Geometry check sheet. Reference: the model listing, model coordinates, mm. A direction names the side the tool comes from. Round coordinates to 2 decimals unless told otherwise and drop trailing zeros. Loops run counter-clockwise (first coordinate to the right, second up) from the corner with the lowest first, then second, coordinate; pieces in that order, holes last. Notation, with made-up numbers: (50, -4) - (103, -4) arc R15 cw to (103, 24) - close; hole circle Ø6 at (-30.75, 88.5). An arc over 180 degrees is marked (long way). Answer in a Markdown table with one row per item. Add a question column.
```python
from build123d import *

# Parameters (mm, degrees)
F3_R = 4.3853298938


with BuildPart() as f1:
    # F0 (on Front) → F1 (revolve)
    with BuildSketch(Plane.XZ):
        Polygon((44.2099806775, 105.9490938586), (45.2899709793, 125.555711587), (44.2724308081, 125.555711587), (37.4149333342, 1.0616940765), (0, 1.0616940765), (0, 0), (35.287540406, 0), (35.287540406, -1.444288413), (38.2944366026, -1.444288413), (40.1810593803, 32.8062891499), (40.531485917, 39.1680862292), (43.8607326026, 99.6086910919), align=None)
    revolve(axis=Axis((0, 0, 69.7766542435), (0, 0, 1)))

    # F4: sweep along a path in F0
    with BuildLine(Plane.XZ) as f4_path:
        add(Plane.XZ * Edge.make_bspline(
            [(44.2099806775, 105.9490938586), (49.0506904174, 105.6739127968), (59.0645866106, 105.0457021821), (72.5638000505, 101.964100219), (76.7064605297, 79.0873827338), (73.2562446897, 42.9019377278), (64.6212325948, 35.2456056894), (45.068033657, 33.5123230208), (41.9423858857, 32.8326484411), (40.1810593803, 32.8062891499)],
            knots=[0, 0, 0, 0, 0.139953431, 0.2625513152, 0.4305704465, 0.6462751927, 0.7639065202, 0.9181752612, 1, 1, 1, 1], degree=3))
    # F3 (on offset) → F4 (sweep)
    with BuildSketch(Plane.XY.offset(79.756)):
        with Locations((75.1930936536, 0)):
            Circle(F3_R)
    sweep(path=f4_path.line)


solid = f1.part
```
Q1. Release check for a two-part mould opening along X. For faces 4 (the cylindrical face through (18.97, 29.755, -0.732)), 5 (the flat face through (9.9, -43.4, 125.556)) record: +X half, -X half, draft (parallel to the pull), parting line (faces both ways), or undercut.
Q2. Scan lines: line 1 (Y direction, x = 0, z = -0.65); line 2 (Z direction, x = -33, y = 0); line 3 (X direction, y = -29, z = 89.5). Record each from-to range of solid material in increasing order. Write a range as from..to.
Q3. Cross-section at B-B, the plane z = 69.5. State how many separate pieces and enclosed holes the cut face has, plus the area to 3 significant figures.
Q4. Set-up check for faces 1 (the flat face through (0, 0, 0)), 2 (the flat face through (-1, 1, 1.062)), 3 (the flat face through (-11, -34, -1.444)): record each of +Z, -Z, +X, -X, +Y, -Y from which the full face is reachable in a straight line by a thin tool's end or side.
Q5. Depth check by flat-ended pin: P1, Ø4, axis at y = -25, z = 53, coming from the +X side; P2, Ø21, axis at x = -4, y = 17, coming from the -Z side; P3, Ø8, axis at y = 4, z = 64, coming from the +X side. Enter the tip coordinate at first touch or a pass-through.
Q6. Cross-section at A-A, the plane z = 20.5. Enter the section's corners in (x, y).
Check sheet entries:
| question | item | result |
|---|---|---|
| 1 | face 4 | undercut |
| 1 | face 5 | draft |
| 2 | line 1 | -38.34..-35.29, 35.29..38.34 |
| 2 | line 2 | 0..1.06 |
| 2 | line 3 | -32.16..-30.78, 30.78..32.16 |
| 3 | separate pieces | 2 |
| 3 | enclosed holes | 1 |
| 3 | area | 327 mm² |
| 4 | face 1 | -Z |
| 4 | face 2 | +Z |
| 4 | face 3 | -Z, +X, -X, +Y, -Y |
| 5 | P1 | x = 34.3 |
| 5 | P2 | z = 0 |
| 5 | P3 | x = 79.29 |
| 6 | outline | circle Ø79.01 at (0, 0); hole circle Ø76.97 at (0, 0) |
